The listing builds one solid part. Answer for the finished solid, in the listing's coordinates (mm). A direction names the side the tool comes from. Give positions to 0.01 mm unless a question says otherwise; leave off trailing zeros. Loops run counter-clockwise (first coordinate to the right, second up) from the corner with the lowest first, then second, coordinate; pieces in that order, holes last. Notation, with made-up numbers: (-11.5, 32) - (-0.5, 32) arc R18 ccw to (-0.5, 50) - close; hole circle Ø1 at (83.5, -16.5). An arc over 180 degrees is marked (long way). Answer in a Markdown table with one row per item. Add a question column.
```python
from build123d import *

# Parameters (mm, degrees)
SKETCH1_W           = 206
SKETCH1_H           = 173
SKETCH1_R           = 1
BOSS_EXTRUDE1_DEPTH = 3


with BuildPart() as part:
    # Sketch1 → Boss-Extrude1 (new body)
    with BuildSketch(Plane(origin=(0, 0, 0), x_dir=(0, 0, -1), z_dir=(1, 0, 0))):
        with Locations((103, 86.5)):
            Rectangle(SKETCH1_W, SKETCH1_H)
        with Locations((204.5, 171.5)):
            Circle(SKETCH1_R, mode=Mode.SUBTRACT)
        with Locations((204.5, 1.5)):
            Circle(SKETCH1_R, mode=Mode.SUBTRACT)
        with Locations((1.5, 171.5)):
            Circle(SKETCH1_R, mode=Mode.SUBTRACT)
        with Locations((1.5, 1.5)):
            Circle(SKETCH1_R, mode=Mode.SUBTRACT)
        with Locations((201.5, 50)):
            Circle(SKETCH1_R, mode=Mode.SUBTRACT)
        with Locations((4.5, 50)):
            Circle(SKETCH1_R, mode=Mode.SUBTRACT)
        with BuildLine():
            Line((30, 158), (176, 158))
            ThreePointArc((176, 158), (183, 151), (176, 144))
            Line((176, 144), (30, 144))
            ThreePointArc((30, 144), (23, 151), (30, 158))
        make_face(mode=Mode.SUBTRACT)
        with BuildLine():
            Line((40, 25), (60, 25))
            ThreePointArc((60, 25), (65, 20), (60, 15))
            Line((60, 15), (40, 15))
            ThreePointArc((40, 15), (35, 20), (40, 25))
        make_face(mode=Mode.SUBTRACT)
        with BuildLine():
            Line((90, 25), (110, 25))
            ThreePointArc((110, 25), (115, 20), (110, 15))
            Line((110, 15), (90, 15))
            ThreePointArc((90, 15), (85, 20), (90, 25))
        make_face(mode=Mode.SUBTRACT)
        with BuildLine():
            Line((146, 25), (166, 25))
            ThreePointArc((166, 25), (171, 20), (166, 15))
            Line((166, 15), (146, 15))
            ThreePointArc((146, 15), (141, 20), (146, 25))
        make_face(mode=Mode.SUBTRACT)
    extrude(amount=BOSS_EXTRUDE1_DEPTH)


solid = part.part
```
(1) A cutting plane is placed at A-A on y = 151. Determine the outline of the cut face in (x, z), plus the area to 3 significant figures.
(2) A tool of negligible diameter and unlimited length cuts with its end or side. For faces 3 (the face through (1, 20, -35)), 4 (the face through (0, 88, -102)), from which of +Z, -Z, +X, -X, +Y, -Y can it reach the whole face along a straight path? Write none if from no direction.
(3) The mould has two halves that part along Y. Classify faces 1 (the face through (3, 88, -102)), 2 (the face through (1, 151, -183)): pulls with the +Y half, pulls with the -Y half, needs draft (parallel to the pull), parting line crosses it, or undercut.
(4) Find the intervals of material crossed by line 1 along Y through (x, z) = (1.7, -156); line 2 along Z through (x, y) = (1.55, 171.5); line 3 along Y through (x, z) = (2.3, -1.5), in increasing order. Write a range as [from, to].
(5) Given pin 1 Ø1.5 at (y, z) = (103, -23.5) entering from -X, flat-ended and moving along its own axis, determine where the tip first touches the part or whether it passes through.
(6) A cutting plane is placed at C-C on y = 20. Determine the outline of the cut face in (x, z).
(7) A cutting plane is placed at D-D on x = 2.4. Give the number of separate pieces and of enclosed holes in the cut face, plus the area to 3 significant figures.
(8) A cutting plane is placed at B-B on z = -122. Determine the outline of the cut face in (x, y), plus the area to 3 significant figures.
Evaluation:
| question | item | result |
|---|---|---|
| 1 | outline | (0, -206) - (3, -206) - (3, -183) - (0, -183) - close; (0, -23) - (3, -23) - (3, 0) - (0, 0) - close |
| 1 | area | 138 mm² |
| 2 | face 3 | +X, -X |
| 2 | face 4 | +Z, -Z, -X, +Y, -Y |
| 3 | face 1 | needs draft |
| 3 | face 2 | undercut |
| 4 | line 1 | y = [0, 15], [25, 144], [158, 173] |
| 4 | line 2 | z = [-206, -205.5], [-203.5, -2.5], [-0.5, 0] |
| 4 | line 3 | y = [0, 0.5], [2.5, 170.5], [172.5, 173] |
| 5 | pin 1 | stops at x = 0 |
| 6 | outline | (0, -206) - (3, -206) - (3, -171) - (0, -171) - close; (0, -141) - (3, -141) - (3, -115) - (0, -115) - close; (0, -85) - (3, -85) - (3, -65) - (0, -65) - close; (0, -35) - (3, -35) - (3, 0) - (0, 0) - close |
| 7 | separate pieces | 1 |
| 7 | enclosed holes | 10 |
| 7 | area | 32,600 mm² |
| 8 | outline | (0, 0) - (3, 0) - (3, 144) - (0, 144) - close; (0, 158) - (3, 158) - (3, 173) - (0, 173) - close |
| 8 | area | 477 mm² |
